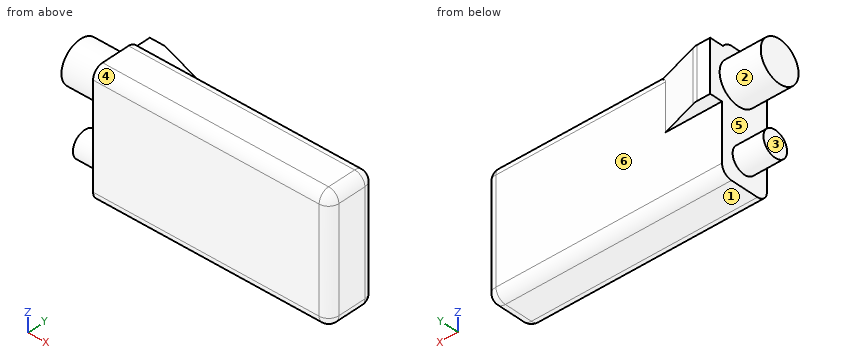
from build123d import *

# Parameters (mm, degrees)
SKETCH_1_W      = 46
SKETCH_1_H      = 24
EXTRUDE_1_DEPTH = 9.5
SKETCH_2_R      = 4
EXTRUDE_2_DEPTH = 8
SKETCH_4_W      = 10
SKETCH_4_H      = 5.984936324
EXTRUDE_3_DEPTH = 3
EXTRUDE_4_DEPTH = 10
SKETCH_6_R      = 2.5
EXTRUDE_5_DEPTH = 6
FILLET_1_R      = 3
FILLET_5_R      = 2
FILLET_6_R      = 2


with BuildPart() as part:
    # 草图1 → 凸台-拉伸1 (new body)
    with BuildSketch(Plane(origin=(0, 0, 0), x_dir=(1, 0, 0), z_dir=(0, 1, 0))):
        Rectangle(SKETCH_1_W, SKETCH_1_H)
    extrude(amount=EXTRUDE_1_DEPTH)

    # 草图2 → 凸台-拉伸2 (add)
    with BuildSketch(Plane.ZY.offset(23)):
        with Locations(Location((6, 6, 0), (0, 0, 118.955024372))):
            Circle(SKETCH_2_R)
    extrude(amount=EXTRUDE_2_DEPTH)

    # 草图4 → 凸台-拉伸3 (add)
    with BuildSketch(Plane.ZY.offset(23)):
        with Locations((6, 9)):
            Rectangle(SKETCH_4_W, SKETCH_4_H)
    extrude(amount=-EXTRUDE_3_DEPTH)

    # 草图5 → 凸台-拉伸4 (add)
    with BuildSketch(Plane.XY.offset(11)):
        Polygon((-20, 11.992468162), (-20, 9.5), (-12, 9.5), align=None)
    extrude(amount=-EXTRUDE_4_DEPTH)

    # 草图6 → 凸台-拉伸5 (add)
    with BuildSketch(Plane.ZY.offset(23)):
        with Locations(Location((-7, 4.749394355, 0), (0, 0, 180))):
            Circle(SKETCH_6_R)
    extrude(amount=EXTRUDE_5_DEPTH)

    # 圆角1
    fillet_1_edges = [part.edges().sort_by_distance(p)[0] for p in [
        (-20, 11.992468162, 6),
    ]]
    fillet(fillet_1_edges, radius=FILLET_1_R)

    # 圆角5
    fillet_5_edges = [part.edges().sort_by_distance(p)[0] for p in [
        (0, 0, 12),
        (0, 0, -12),
        (0, 9.5, -12),
        (0, 9.5, 12),
    ]]
    fillet(fillet_5_edges, radius=FILLET_5_R)

    # 圆角6
    fillet_6_edges = [part.edges().sort_by_distance(p)[0] for p in [
        (23, 4.75, 12),
        (23, 0, 0),
        (23, 4.75, -12),
        (23, 9.5, 0),
        (23, 8.914213562, 11.414213562),
        (23, 8.914213562, -11.414213562),
        (23, 0.585786438, -11.414213562),
        (23, 0.585786438, 11.414213562),
    ]]
    fillet(fillet_6_edges, radius=FILLET_6_R)


solid = part.part
Geometry check sheet. Reference: the model listing, model coordinates, mm. Face numbers are marked on the shaded views. A direction names the side the tool comes from. Round coordinates to 2 decimals unless told otherwise and drop trailing zeros. Order: outer loops, then holes, each group sorted by start corner. A loop starts at its lowest first (then second) coordinate and runs counter-clockwise, first axis right, second up. Notation, with made-up numbers: M 67.5,25 L 107.5,25 A20 cw 107.5,47 Z; hole C 39.5,73 d4. An arc over 180 degrees is marked long. Write each question's results on one line, items separated by ' | '. Start each with the question number.
1. Set-up check for the marked faces 4, 5 and 6: record each of +Z, -Z, +X, -X, +Y, -Y from which the full face is reachable in a straight line by a thin tool's end or side.
2. Cross-section at A-A on z = 6. Record the boundary of the cut face in (x, y), plus the area to 3 significant figures.
3. Cross-section at B-B on x = -3. Record the boundary of the cut face in (y, z), plus the area to 3 significant figures.
4. Go/stop test with flat-tipped pins: P1, Ø1, axis at x = -2.5, z = 7.5, coming from the +Y side; P2, Ø2, axis at x = -15.5, y = 11.5, coming from the -Z side; P3, Ø2.5, axis at y = 5, z = -6.5, coming from the -X side. Record where each tip stops, or that it passes through.
5. Cross-section at D-D on z = -7. Record the boundary of the cut face in (x, y).
6. Cross-section at C-C on y = 3.25. Record the boundary of the cut face in (x, z).
7. Material ranges on L1, parallel to Y at x = -9, z = -3.75; L2, parallel to X at y = 5.25, z = -10; L3, parallel to Z at x = -22.5, y = 10, recorded low to high. Write a range as from..to.
8. Draft check along Z on the marked faces 1, 2 and 3. Enter one of: pulls with the +Z half, pulls with the -Z half, needs draft (parallel to the pull), parting line crosses it, or undercut.
Resolved:
1) face 4: +Z, +X, -X, -Y | face 5: -X | face 6: -Z, +X, +Y
2) outline: M -31,2 L -23,2 L -23,0 L 21,0 A2 ccw 23,2 L 23,7.5 A2 ccw 21,9.5 L -12,9.5 L -19.56,11.86 A3 ccw -20.46,11.99 L -23,11.99 L -23,10 L -31,10 Z | area: 517 mm2
3) outline: M 0,-10 A2 ccw 2,-12 L 7.5,-12 A2 ccw 9.5,-10 L 9.5,10 A2 ccw 7.5,12 L 2,12 A2 ccw 0,10 Z | area: 225 mm2
4) P1: y = 9.5 | P2: z = 1 | P3: x = -29
5) outline: M -29,2.25 L -23,2.25 L -23,0 L 21,0 A2 ccw 23,2 L 23,7.5 A2 ccw 21,9.5 L -23,9.5 L -23,7.25 L -29,7.25 Z
6) outline: M -31,3.1 L -23,3.1 L -23,-5 L -29,-5 L -29,-9 L -23,-9 L -23,-12 L 21,-12 A2 ccw 23,-10 L 23,10 A2 ccw 21,12 L -23,12 L -23,8.9 L -31,8.9 Z
7) L1: 0..9.5 | L2: -23..23 | L3: 1..11
8) face 1: pulls with the -Z half | face 2: undercut | face 3: needs draft
